Autodesk Inventor part; units mm, degrees
ref_plane "YZ Plane" through (0, 0, 0) normal (1, 0, 0) x (0, 1, 0)
ref_plane "XZ Plane" through (0, 0, 0) normal (0, 1, 0) x (-1, 0, 0)
ref_plane "XY Plane" through (0, 0, 0) normal (0, 0, 1) x (1, 0, 0)
sketch "Boceto1" plane through (0, 0, 0) normal (0, 0, 1) x (1, 0, 0)
  line L0 (-4.2, 2) -> (4.2, 2)
  line L1 (-4.4, 4.8) -> (-4.4, 2.2)
  line L2 (4.2, 5) -> (-4.2, 5)
  line L3 (4.4, 2.2) -> (4.4, 4.8)
  line L4 (6, 6.2) -> (6, 0.2)
  line L5 (-3, 6.2) -> (1.6383, 6.2)
  line L6 (-6, 0.2) -> (-6, 6)
  line L7 (-5.8, 0) -> (5.8, 0)
  line L8 (-5.8, 28.2) -> (5.8, 28.2)
  line L9 (6, 28) -> (6, 26.4)
  line L10 (5.8, 26.2) -> (-1.6383, 26.2)
  line L11 (-6, 26.1436) -> (-6, 28)
  line L12 (-3, 6.2) -> (-5.8, 6.2)
  line L13 (-5.1901, 10.47) -> (-5.0521, 10.516)
  line L14 (5.1901, 14.47) -> (5.0521, 14.516)
  line L15 (1.7647, 6.9795) -> (-5.622, 9.441)
  line L16 (-7.7794, 10.1599) -> (-7.7493, 10.2501)
  line L17 (7.7794, 6.2401) -> (7.4, 5.1016)
  line L18 (-5.622, 10.959) -> (2.9651, 13.8205)
  line L19 (7.7493, 14.2501) -> (7.7794, 14.1599)
  line L20 (-7.7493, 10.1499) -> (-7.7794, 10.2401)
  line L21 (2.9651, 14.5795) -> (-5.622, 17.441)
  line L22 (-7.7794, 18.1599) -> (-7.7493, 18.2501)
  line L23 (-2.9651, 17.8205) -> (5.622, 14.959)
  line L24 (7.7794, 14.2401) -> (7.7493, 14.1499)
  line L25 (-2.9651, 18.5795) -> (5.622, 21.441)
  line L26 (7.7794, 22.1599) -> (7.7493, 22.2501)
  line L27 (-7.7794, 18.2401) -> (-7.7493, 18.1499)
  line L28 (-1.7647, 25.4205) -> (5.622, 22.959)
  line L29 (7.7794, 22.2401) -> (7.7493, 22.1499)
  line L30 (6.0017, 22.8324) -> (6, 22.8319)
  line L31 (2.9651, 21.8205) -> (-5.622, 18.959)
  line L32 (6.0017, 21.5676) -> (6, 21.5681)
  line L33 (2.9651, 22.5795) -> (-5.4529, 25.3847)
  line L34 (-2.9651, 9.8205) -> (5.4529, 7.0153)
  line L35 (5.622, 13.441) -> (-2.9651, 10.5795)
  line L36 (-6, 9.5681) -> (-6.0017, 9.5676)
  line L37 (-6.0017, 10.8324) -> (-6, 10.8319)
  line L38 (-5.2246, 10.5735) -> (-5.0521, 10.516)
  line L39 (6, 6.2564) -> (6, 6.2)
  arc A0 (5.622, 21.441) -> (5.622, 22.959) centre (5.3691, 22.2) ccw
  arc A1 (-5.622, 18.959) -> (-5.622, 17.441) centre (-5.3691, 18.2) ccw
  arc A2 (5.622, 13.441) -> (5.622, 14.959) centre (5.3691, 14.2) ccw
  arc A3 (-5.622, 10.959) -> (-5.622, 9.441) centre (-5.3691, 10.2) ccw
  arc A4 (6, 6.2564) -> (5.4529, 7.0153) centre (5.2, 6.2564) ccw
  arc A5 (-6, 26.1436) -> (-5.4529, 25.3847) centre (-5.2, 26.1436) ccw
  arc A6 (-2.8711, 26.2) -> (-2.9343, 25.8103) centre (-2.8711, 26) ccw
  arc A7 (-3.5345, 18.3897) -> (-3.5345, 18.0103) centre (-3.4713, 18.2) ccw
  arc A8 (3.5345, 14.0103) -> (3.5345, 14.3897) centre (3.4713, 14.2) ccw
  arc A9 (-3.5345, 10.3897) -> (-3.5345, 10.0103) centre (-3.4713, 10.2) ccw
  arc A10 (2.8711, 6.2) -> (2.9343, 6.5897) centre (2.8711, 6.4) ccw
  arc A11 (-5.8, 6.2) -> (-6, 6) centre (-5.8, 6) ccw
  arc A12 (-6, 0.2) -> (-5.8, 0) centre (-5.8, 0.2) ccw
  arc A13 (5.8, 0) -> (6, 0.2) centre (5.8, 0.2) ccw
  arc A14 (-5.8, 28.2) -> (-6, 28) centre (-5.8, 28) ccw
  arc A15 (6, 28) -> (5.8, 28.2) centre (5.8, 28) ccw
  arc A16 (5.8, 26.2) -> (6, 26.4) centre (5.8, 26.4) ccw
  arc A17 (-4.2, 5) -> (-4.4, 4.8) centre (-4.2, 4.8) ccw
  arc A18 (-4.4, 2.2) -> (-4.2, 2) centre (-4.2, 2.2) ccw
  arc A19 (4.2, 2) -> (4.4, 2.2) centre (4.2, 2.2) ccw
  arc A20 (4.4, 4.8) -> (4.2, 5) centre (4.2, 4.8) ccw
  arc A21 (3.5345, 22.0103) -> (3.5345, 22.3897) centre (3.4713, 22.2) ccw
  arc A22 (2.9651, 21.8205) -> (2.9651, 22.5795) centre (2.8386, 22.2) ccw
  arc A23 (-2.9651, 18.5795) -> (-2.9651, 17.8205) centre (-2.8386, 18.2) ccw
  arc A24 (2.9651, 13.8205) -> (2.9651, 14.5795) centre (2.8386, 14.2) ccw
  arc A25 (-2.9651, 10.5795) -> (-2.9651, 9.8205) centre (-2.8386, 10.2) ccw
  arc A26 (1.6383, 6.2) -> (1.7647, 6.9795) centre (1.6383, 6.6) ccw
  arc A27 (-1.6383, 26.2) -> (-1.7647, 25.4205) centre (-1.6383, 25.8) ccw
  point P0 (0, 0)
  point P1 (0, 0)
  point P2 (6, 26.2)
  point P3 (6, 28.2)
  point P4 (6, 14.2)
  point P5 (6, 18.2)
  point P6 (6, 22.2)
  point P7 (-6, 10.2)
  point P8 (-6, 14.2)
  point P9 (-6, 18.2)
  point P10 (-6, 22.2)
  point P11 (0, 8.2)
  point P12 (0, 12.2)
  point P13 (0, 16.2)
  point P14 (0, 20.2)
  point P15 (0, 24.2)
  point P16 (4.1039, 22.2)
  dimension "d0" = 2
  dimension "d7" = 16
  dimension "d22" = 0.8
  dimension "d23" = 0.2
  dimension "d24" = 0.2
  dimension "d30" = 0.2
  dimension "d31" = 0.4
extrude "Extrusión1" add sketch "Boceto1" along normal mid plane 12
sketch "Boceto2" plane through (0, 0, 0) normal (0, 1, 0) x (-1, 0, 0)
  circle A0 centre (0, 0) radius 2
  dimension "d27" = 4
extrude "Extrusión2" cut sketch "Boceto2" along normal blind 40
properties part number "_3DPrint"
Can you work these out from the model? Positions are in its coordinate system, mm. A direction names the side the tool comes from. Give positions to 0.01 mm unless a question says otherwise; leave off trailing zeros. Order: outer loops, then holes, each group sorted by start corner. A loop starts at its lowest first (then second) coordinate and runs counter-clockwise, first axis right, second up. Notation, with made-up numbers: M 42.25,8 L 71.25,8 A13 ccw 71.25,16 Z; hole C 22.25,-22.5 d4. An arc over 180 degrees is marked long. Write item = value, one per line. Start each with the question number.
Q1. Suppose I cut it at A-A (y = 3). Write out the boundary of the cut face in (x, z).
Q2. For faces 5 (the flat face through (-2.12, 24.274, -1.417)), 6 (the flat face through (2.2, 20.3, -0.1)), 7 (the flat face through (2, 5, -1)), 8 (the flat face through (-6, 3, 0)), which set-ups out of +Z, -Z, +X, -X, +Y, -Y let a thin tool reach every point of the face, with its end or its side?
Q3. We'd pull the mould along X, two halves only. Please class faces 1 (the flat face through (4.4, 3, 0)), 2 (the flat face through (-3, 0, 0)), 3 (the flat face through (-6, 27, 0)), 4 (the flat face through (-4.4, 4, 0)): pulls with the +X half, pulls with the -X half, needs draft (parallel to the pull), parting line crosses it, or undercut.
Q4. Suppose I cut it at C-C (x = 0). Count the separate pieces of the cut face and the enclosed holes in it, plus the area to 3 significant figures.
Q5. I need wall thicknesses on probe 1 along Z at (x, y) = (0, 20.7); probe 2 along Y at (x, z) = (3.5, 3.75); probe 3 along Y at (x, z) = (5.25, -4). Which ranges of each line are inside material? Lowest first, please. Write a range as [from, to].
Q6. Will these pins go through, and if not, where does the flat tip stop? pin 1 Ø2.5 at (x, z) = (0, 0) entering from +Y; pin 2 Ø0.8 at (y, z) = (3, 2.5) entering from -X; pin 3 Ø1.8 at (y, z) = (27.5, -1) entering from +X.
Q7. Suppose I cut it at B-B (x = 4.75). Write out the boundary of the cut face in (y, z), plus the area to 3 significant figures.
Check result:
q1.outline = M -6,-6 L -4.4,-6 L -4.4,6 L -6,6 Z; M 4.4,-6 L 6,-6 L 6,6 L 4.4,6 Z
q2.face_5 = +Z, -Z, -X
q2.face_6 = +Z, -Z, +X
q2.face_7 = +Z, -Z
q2.face_8 = +Z, -Z, -X, -Y
q3.face_1 = undercut
q3.face_2 = needs draft
q3.face_3 = pulls with the -X half
q3.face_4 = undercut
q4.separate_pieces = 16
q4.enclosed_holes = 0
q4.area = 92.2 mm2
q5.probe_1 = [-6, -2], [2, 6]
q5.probe_2 = [0, 2], [5, 7.67], [12.73, 15.67], [20.73, 23.67], [26.2, 28.2]
q5.probe_3 = [0, 7.08], [13.32, 15.08], [21.32, 23.08], [26.2, 28.2]
q6.pin_1 = through
q6.pin_2 = -6
q6.pin_3 = 6
q7.outline = M 0,-6 L 7.25,-6 L 7.25,6 L 0,6 Z; M 13.15,-6 L 15.25,-6 L 15.25,6 L 13.15,6 Z; M 21.15,-6 L 23.25,-6 L 23.25,6 L 21.15,6 Z; M 26.2,-6 L 28.2,-6 L 28.2,6 L 26.2,6 Z
q7.area = 161 mm2
